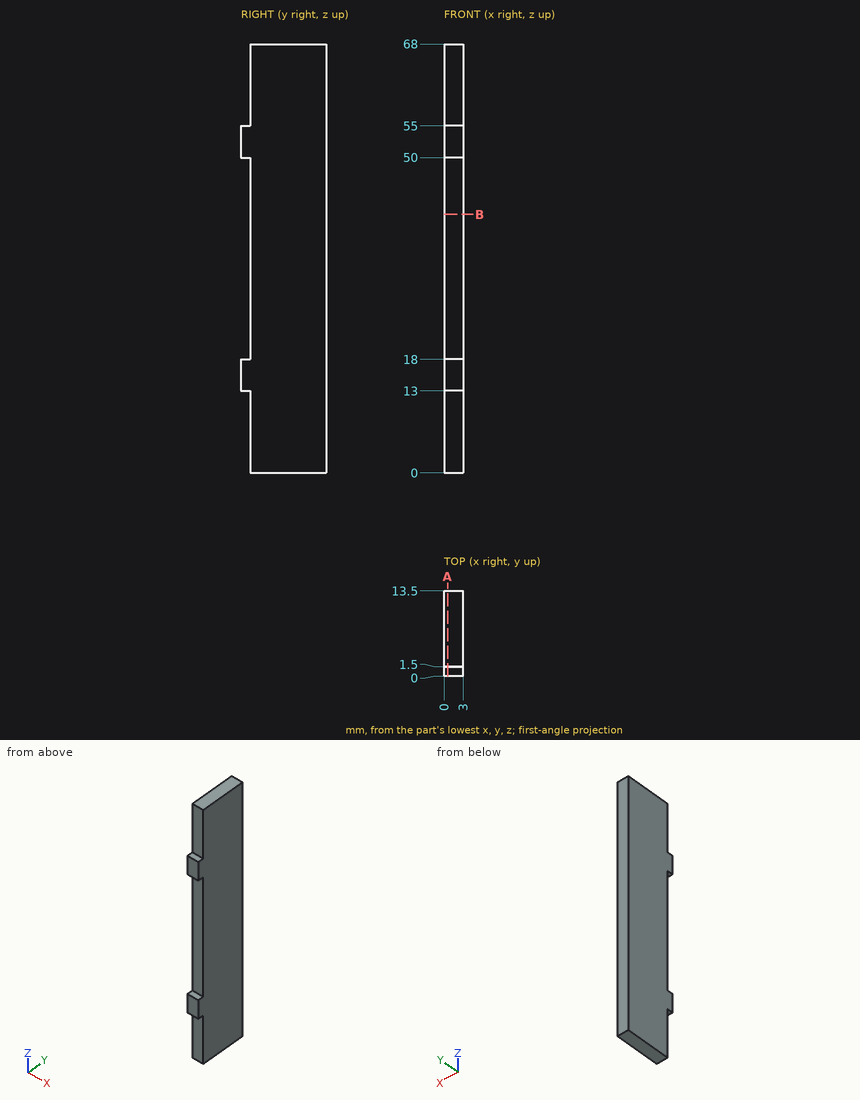
Part print with two shaded views. Sizes in mm from the minimum x, y, z corner. Round coordinates to 2 decimals unless told otherwise and drop trailing zeros. Write each loop counter-clockwise with the first axis right and the second up, starting at its lowest first coordinate (ties: lowest second). Pieces come first, ordered by that corner, then holes. Notation, with made-up numbers: (-37.75, 17.25) -> (-32.75, 17.25) arc R18 cw to (-32.75, 43.25) -> close; hole circle Ø1 at (40.5, -4.75). An arc over 180 degrees is marked (long way). Put each result on its own line as item: value.
Item 1: Flat gauge pins, fed straight in: P1, Ø1.5, axis at x = 2.5, z = 59, coming from the -Y side; P2, Ø0.8, axis at x = 1, y = 0.5, coming from the +Z side; P3, Ø1.6, axis at x = 2, y = 0.5, coming from the -Z side. Where does each tip first touch, or does it go through?
Here are the results:
P1: stops at y = 1.5
P2: stops at z = 55
P3: stops at z = 13
Item 2: Slice it at B-B, the plane z = 41. Give the cut face in (x, y).
Here are the results:
outline: (0, 1.5) -> (3, 1.5) -> (3, 13.5) -> (0, 13.5) -> close
Item 3: Slice it at A-A, the plane x = 0.55. Give the cut face in (y, z), plus the area to 3 significant figures.
Here are the results:
outline: (0, 13) -> (1.5, 13) -> (1.5, 0) -> (13.5, 0) -> (13.5, 68) -> (1.5, 68) -> (1.5, 55) -> (0, 55) -> (0, 50) -> (1.5, 50) -> (1.5, 18) -> (0, 18) -> close
area: 831 mm^2
Item 4: Wall check: probe 1 along Y at (x, z) = (2.3, 24.5). Give the ranges that are in metal, low to high. Write a range as from..to.
Here are the results:
probe 1: y = 1.5..13.5
